from build123d import *

# Parameters (mm, degrees)
F1_DEPTH = 95.25
F2_R     = 1.98374
F3_R     = 3.69316
F4_R     = 0.762
F5_R     = 1.8288
F6_DEPTH = 1.70942
F7_R     = 10.751496
F7_R_2   = 1.5
F8_DEPTH = 1.70942


with BuildPart() as f1:
    # F0 (on Top) → F1 (new body)
    with BuildSketch(Plane.XY):
        Polygon((0, -13.29058), (0, 0), (45.08116, 0), (45.08116, -13.29058), (61.79058, -13.29058), (61.79058, -11.58116), (46.79058, -11.58116), (46.79058, 1.70942), (-1.70942, 1.70942), (-1.70942, -11.58116), (-16.70942, -11.58116), (-16.70942, -13.29058), align=None)
    extrude(amount=F1_DEPTH)

    # F2
    f2_edges = [f1.edges().sort_by_distance(p)[0] for p in [
        (0, 0, 47.625),
        (-1.70942, -11.58116, 47.625),
        (45.08116, 0, 47.625),
        (46.79058, -11.58116, 47.625),
    ]]
    fillet(f2_edges, radius=F2_R)

    # F3
    f3_edges = [f1.edges().sort_by_distance(p)[0] for p in [
        (0, -13.29058, 47.625),
        (-1.70942, 1.70942, 47.625),
        (46.79058, 1.70942, 47.625),
        (45.08116, -13.29058, 47.625),
    ]]
    fillet(f3_edges, radius=F3_R)

    # F4
    f4_edges = [f1.edges().sort_by_distance(p)[0] for p in [
        (-16.70942, -12.43587, 0),
        (-16.70942, -12.43587, 95.25),
        (61.79058, -12.43587, 0),
        (61.79058, -12.43587, 95.25),
    ]]
    fillet(f4_edges, radius=F4_R)

    # F5 (on face) → F6 (cut, through all)
    with BuildSketch(Plane.XZ):
        with Locations((5.15874, 92.075)):
            Circle(F5_R)
        with Locations((5.15874, 3.175)):
            Circle(F5_R)
        with Locations((39.92242, 92.075)):
            Circle(F5_R)
        with Locations((39.92242, 3.175)):
            Circle(F5_R)
    extrude(amount=-F6_DEPTH, mode=Mode.SUBTRACT)

    # F7 (on face) → F8 (cut, through all)
    with BuildSketch(Plane.XZ):
        with Locations((22.54058, 66.603258)):
            Circle(F7_R)
        with Locations((38.040574, 82.103252)):
            Circle(F7_R_2)
        with Locations((38.040574, 51.103263)):
            Circle(F7_R_2)
        with Locations((7.040586, 51.103263)):
            Circle(F7_R_2)
        with Locations((7.040586, 82.103252)):
            Circle(F7_R_2)
    extrude(amount=-F8_DEPTH, mode=Mode.SUBTRACT)


solid = f1.part
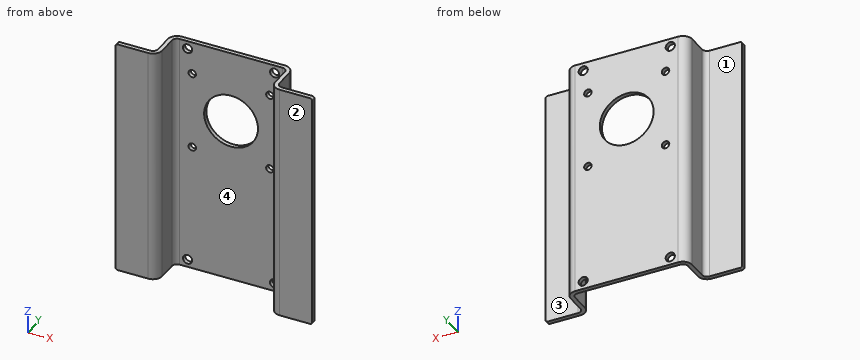
Verification items for the finished model (mm, model axes). Face numbers are marked on the shaded views. A direction names the side the tool comes from. Coordinates: 2 decimals unless noted, no trailing zeros. Loops run counter-clockwise (first coordinate to the right, second up) from the corner with the lowest first, then second, coordinate; pieces in that order, holes last. Notation, with made-up numbers: (2.5, 8) -> (12.5, 8) arc R35 cw to (12.5, 43) -> close; hole circle Ø10 at (19.5, 6). An arc over 180 degrees is marked (long way). Answer as a JSON object with one key per item and string values. Group by question number.
Item 1: Depth check by flat-ended pin: pin 1 (6.5 mm diameter, centred on x = -7.5, z = 65, fed in from +Y); pin 2 (4 mm diameter, centred on y = -7, z = 47, fed in from +X); pin 3 (1.8 mm diameter, centred on x = 38.04, z = 82.1, fed in from +Y); pin 4 (2.5 mm diameter, centred on y = -5.5, z = 36.5, fed in from -X). Enter the tip coordinate at first touch or a pass-through.
Item 2: Scan lines: probe 1 along X at (y, z) = (-9.25, 68); probe 2 along Y at (x, z) = (58, 88); probe 3 along Y at (x, z) = (20, 86). Record each from-to range of solid material in increasing order.
Item 3: Tool access check on the marked faces 1 and 2. Record the directions out of +Z, -Z, +X, -X, +Y, -Y that give a thin tool (end or side, any length) a straight path to the whole face; none if there is none.
Item 4: Sectioned sample at C-C on z = 60. Record the boundary of the cut face in (x, y).
Item 5: Sectioned sample at D-D on z = 31. Record the boundary of the cut face in (x, y), plus the area to 3 significant figures.
Item 6: Sectioned sample at B-B on x = 24. Record the boundary of the cut face in (y, z).
Item 7: Mould release check, pull along Y, two halves, no side actions. Record for the marked faces 3 and 4: +Y half, -Y half, draft (parallel to the pull), parting line (faces both ways), or undercut.
Item 8: Sectioned sample at A-A on y = -7.5. Record the boundary of the cut face in (x, z), plus the area to 3 significant figures.
Evaluation:
{
 "1": {"pin 1": "stops at y = -11.58", "pin 2": "stops at x = 46.79", "pin 3": "passes through", "pin 4": "stops at x = -1.71"},
 "2": {"probe 1": "x = -1.71 to 0, 45.08 to 46.79", "probe 2": "y = -13.29 to -11.58", "probe 3": "y = 0 to 1.71"},
 "3": {"face 1": "+Z, -Z, -X, +Y", "face 2": "+Z, -Z, +X, -X, -Y"},
 "4": {"outline": "(-16.71, -13.29) -> (-3.69, -13.29) arc R3.69 ccw to (0, -9.6) -> (0, -1.98) arc R1.98 cw to (1.98, 0) -> (14.06, 0) -> (14.06, 1.71) -> (1.98, 1.71) arc R3.69 ccw to (-1.71, -1.98) -> (-1.71, -9.6) arc R1.98 cw to (-3.69, -11.58) -> (-16.71, -11.58) -> close; (31.03, 0) -> (43.1, 0) arc R1.98 cw to (45.08, -1.98) -> (45.08, -9.6) arc R3.69 ccw to (48.77, -13.29) -> (61.79, -13.29) -> (61.79, -11.58) -> (48.77, -11.58) arc R1.98 cw to (46.79, -9.6) -> (46.79, -1.98) arc R3.69 ccw to (43.1, 1.71) -> (31.03, 1.71) -> close"},
 "5": {"outline": "(-16.71, -13.29) -> (-3.69, -13.29) arc R3.69 ccw to (0, -9.6) -> (0, -1.98) arc R1.98 cw to (1.98, 0) -> (43.1, 0) arc R1.98 cw to (45.08, -1.98) -> (45.08, -9.6) arc R3.69 ccw to (48.77, -13.29) -> (61.79, -13.29) -> (61.79, -11.58) -> (48.77, -11.58) arc R1.98 cw to (46.79, -9.6) -> (46.79, -1.98) arc R3.69 ccw to (43.1, 1.71) -> (1.98, 1.71) arc R3.69 ccw to (-1.71, -1.98) -> (-1.71, -9.6) arc R1.98 cw to (-3.69, -11.58) -> (-16.71, -11.58) -> close", "area": "171 mm²"},
 "6": {"outline": "(0, 0) -> (1.71, 0) -> (1.71, 55.95) -> (0, 55.95) -> close; (0, 77.26) -> (1.71, 77.26) -> (1.71, 95.25) -> (0, 95.25) -> close"},
 "7": {"face 3": "+Y half", "face 4": "-Y half"},
 "8": {"outline": "(-1.71, 0) -> (0, 0) -> (0, 95.25) -> (-1.71, 95.25) -> close; (45.08, 0) -> (46.79, 0) -> (46.79, 95.25) -> (45.08, 95.25) -> close", "area": "326 mm²"}
}
